Build history of the part. All positions in model axes, mm. A direction names the side the tool comes from. Coordinates: 2 decimals unless noted, no trailing zeros. Loops run counter-clockwise (first coordinate to the right, second up) from the corner with the lowest first, then second, coordinate; pieces in that order, holes last.
Item 1: Cut at C-C (x = -15.5). List the corners of the cut face in (y, z), and give its area (3 significant figures).
Item 2: Flat gauge pins, fed straight in: pin 1 (3 mm diameter, centred on x = 14, z = 8.5, fed in from +Y); pin 2 (2.5 mm diameter, centred on x = 36.5, y = -26.5, fed in from +Z); pin 3 (1.5 mm diameter, centred on x = 22, z = 14, fed in from -Y); pin 4 (4.5 mm diameter, centred on y = -2.5, z = 12.5, fed in from +X). Where does each tip first touch, or does it go through?
Item 3: Cut at A-A (y = -26.5). List the corners of the cut face in (x, z), and give its area (3 significant figures).
Item 4: Mould opens along X. For faces 1 (the face through (35, 0, 9)), 2 (the face through (35.284, -25.385, 0.838)), 3 (the face through (0, 25, 9)) say: released by +X, released by -X, zero draft, split by the parting line, or undercut.
Item 5: Cut at D-D (z = 3.5). List the corners of the cut face in (x, y), and give its area (3 significant figures).
Item 6: Drill centre lines: line 1 along Y through (x, z) = (-36.5, 0.8); line 2 along X through (y, z) = (-5, 5.25); line 3 along Y through (x, z) = (-21.5, 7.75). Where is each one in solid material? Low to high.
Item 7: Cut at B-B (x = 36.5). List the corners of the cut face in (y, z).
Item 8: 3-axis set-ups, long thin cutter, end or side, ignore diameter. For faces 4 (the face through (0, -25, 9)), 5 (the face through (-35, 0, 9)), 6 (the face through (-1, -29, 1)): which of +Z, -Z, +X, -X, +Y, -Y reach the whole face in a straight line?
from build123d import *

# Parameters (mm, degrees)
ESBO_O1_W                = 78
ESBO_O1_H                = 58
ESBO_O1_R                = 1.65
RESSALTO_EXTRUS_O1_DEPTH = 1.7
ESBO_O2_W                = 70
ESBO_O2_H                = 50
RESSALTO_EXTRUS_O2_DEPTH = 15


with BuildPart() as part:
    # Esboço1 → Ressalto-extrusão1 (new body)
    with BuildSketch(Plane.XY):
        Rectangle(ESBO_O1_W, ESBO_O1_H)
        with Locations((-36.5, 26.5)):
            Circle(ESBO_O1_R, mode=Mode.SUBTRACT)
        with Locations(Location((-36.5, -26.5, 0), (0, 0, 180))):
            Circle(ESBO_O1_R, mode=Mode.SUBTRACT)
        with Locations(Location((36.5, 26.5, 0), (0, 0, 180))):
            Circle(ESBO_O1_R, mode=Mode.SUBTRACT)
        with Locations((36.5, -26.5)):
            Circle(ESBO_O1_R, mode=Mode.SUBTRACT)
    extrude(amount=RESSALTO_EXTRUS_O1_DEPTH)

    # Esboço2 → Ressalto-extrusão2 (add)
    with BuildSketch(Plane.XY.offset(1.7)):
        Rectangle(ESBO_O2_W, ESBO_O2_H)
    extrude(amount=RESSALTO_EXTRUS_O2_DEPTH)


solid = part.part
Filled sheet:
1. outline: (-29, 0) - (29, 0) - (29, 1.7) - (25, 1.7) - (25, 16.7) - (-25, 16.7) - (-25, 1.7) - (-29, 1.7) - close
1. area: 849 mm2
2. pin 1: stops at y = 25
2. pin 2: passes through
2. pin 3: stops at y = -25
2. pin 4: stops at x = 35
3. outline: (-39, 0) - (-38.15, 0) - (-38.15, 1.7) - (-39, 1.7) - close; (-34.85, 0) - (34.85, 0) - (34.85, 1.7) - (-34.85, 1.7) - close; (38.15, 0) - (39, 0) - (39, 1.7) - (38.15, 1.7) - close
3. area: 121 mm2
4. face 1: released by +X
4. face 2: undercut
4. face 3: zero draft
5. outline: (-35, -25) - (35, -25) - (35, 25) - (-35, 25) - close
5. area: 3,500 mm2
6. line 1: y = -29 to -28.15, -24.85 to 24.85, 28.15 to 29
6. line 2: x = -35 to 35
6. line 3: y = -25 to 25
7. outline: (-29, 0) - (-28.15, 0) - (-28.15, 1.7) - (-29, 1.7) - close; (-24.85, 0) - (24.85, 0) - (24.85, 1.7) - (-24.85, 1.7) - close; (28.15, 0) - (29, 0) - (29, 1.7) - (28.15, 1.7) - close
8. face 4: +Z, +X, -X, -Y
8. face 5: +Z, -X, +Y, -Y
8. face 6: +Z, -Z, +X, -X, -Y
